from build123d import *

# Parameters (mm, degrees)
SKETCH_3_R               = 275
SKETCH_3_R_2             = 185
SKETCH_3_R_3             = 27
SKETCH_3_R_4             = 18
EXTRUDE_1_DEPTH          = 12
CUT_EXTRUDE_2_DEPTH      = 12
CUT_EXTRUDE_2_DEPTH_BACK = 390.093819021
SKETCH_4_R               = 18


with BuildPart() as part:
    # 草图3 → 凸台-拉伸1 (new body)
    with BuildSketch(Plane(origin=(0, 0, 0), x_dir=(1, 0, 0), z_dir=(0, 1, 0))):
        with Locations(Location((0, 0, 0), (0, 0, 270))):
            Circle(SKETCH_3_R)
        with Locations(Location((0, 0, 0), (0, 0, 270))):
            Circle(SKETCH_3_R_2, mode=Mode.SUBTRACT)
        with Locations(Location((240, 0, 0), (0, 0, 270))):
            Circle(SKETCH_3_R_3, mode=Mode.SUBTRACT)
        with Locations(Location((234.2578125, -52.185029297, 0), (0, 0, 270))):
            Circle(SKETCH_3_R_4, mode=Mode.SUBTRACT)
        with Locations(Location((-120, -207.846096908, 0), (0, 0, 270))):
            Circle(SKETCH_3_R_3, mode=Mode.SUBTRACT)
        with Locations(Location((-120, 207.846096908, 0), (0, 0, 270))):
            Circle(SKETCH_3_R_3, mode=Mode.SUBTRACT)
        with Locations(Location((-71.935345182, 228.965731308, 0), (0, 0, 270))):
            Circle(SKETCH_3_R_4, mode=Mode.SUBTRACT)
        with Locations(Location((-162.322467318, -176.780702012, 0), (0, 0, 270))):
            Circle(SKETCH_3_R_4, mode=Mode.SUBTRACT)
    extrude(amount=EXTRUDE_1_DEPTH)

    # 草图4 → 切除-拉伸2 (cut, two sides: drawn at the far end of the back side and taken through both)
    with BuildSketch(Plane(origin=(0, 0, 0), x_dir=(1, 0, 0), z_dir=(0, 1, 0)).offset(-CUT_EXTRUDE_2_DEPTH_BACK)):
        with Locations(Location((-228, 0, 0), (0, 0, 270))):
            Circle(SKETCH_4_R)
        with Locations(Location((114, 197.453792063, 0), (0, 0, 270))):
            Circle(SKETCH_4_R)
        with Locations(Location((114, -197.453792063, 0), (0, 0, 270))):
            Circle(SKETCH_4_R)
    extrude(amount=CUT_EXTRUDE_2_DEPTH + CUT_EXTRUDE_2_DEPTH_BACK, mode=Mode.SUBTRACT)


solid = part.part
Source: CAD feature listing. Evaluate the final solid. Frame: model axes, mm. Coordinates: 2 decimals unless noted, no trailing zeros. Loops run counter-clockwise (first coordinate to the right, second up) from the corner with the lowest first, then second, coordinate; pieces in that order, holes last. Notation, with made-up numbers: (28, 51.5) - (56, 51.5) arc R13 ccw to (56, 68.5) - close; hole circle Ø4 at (34, -14). An arc over 180 degrees is marked (long way). One line per item, written item: value. Start each with the question number.
1. Section B-B (z = 0). Return the cut outline in (x, y).
2. Mould query, pull axis Z, two halves, no side actions, for faces 1 (the flat face through (-57, 0, 179)), 2 (the cylindrical face through (82.6, 5.9, 262.3)), 3 (the cylindrical face through (-71.14, 5.92, -246.95)). Classes: pulls with the +Z half, pulls with the -Z half, needs draft (parallel to the pull), parting line crosses it, or undercut.
3. Section C-C (x = -120). Return the cut outline in (y, z), and give its area (3 significant figures).
4. Section A-A (x = 0). Return the cut outline in (y, z), and give its area (3 significant figures).
5. Section D-D (z = -160.5). Return the cut outline in (x, y), and give its area (3 significant figures).
6. Contact query for flat-ended pins moving along their axis: P1, Ø4, axis at x = -215.5, y = 6.5, coming from the +Z side; P2, Ø21.5, axis at x = -228, z = 0, coming from the +Y side; P3, Ø1, axis at x = 27.5, y = 10.5, coming from the -Z side; P4, Ø1.5, axis at y = 5, z = 4.5, coming from the +X side. Output: stop coordinate, or through.
7. Ray query, L1, parallel to X at y = 2.5, z = 0; L2, parallel to Z at x = 127.5, y = 9; L3, parallel to X at y = 7.75, z = -201. Return the intervals inside material, ascending.
Verdict:
1. outline: (-275, 0) - (-246, 0) - (-246, 12) - (-275, 12) - close; (-210, 0) - (-185, 0) - (-185, 12) - (-210, 12) - close; (185, 0) - (213, 0) - (213, 12) - (185, 12) - close; (267, 0) - (275, 0) - (275, 12) - (267, 12) - close
2. face 1: needs draft
2. face 2: parting line crosses it
2. face 3: undercut
3. outline: (0, -247.44) - (12, -247.44) - (12, -234.85) - (0, -234.85) - close; (0, -180.85) - (12, -180.85) - (12, -140.8) - (0, -140.8) - close; (0, 140.8) - (12, 140.8) - (12, 180.85) - (0, 180.85) - close; (0, 234.85) - (12, 234.85) - (12, 247.44) - (0, 247.44) - close
3. area: 1,260 mm2
4. outline: (0, -275) - (12, -275) - (12, -185) - (0, -185) - close; (0, 185) - (12, 185) - (12, 275) - (0, 275) - close
4. area: 2,160 mm2
5. outline: (-223.3, 0) - (-92, 0) - (-92, 12) - (-223.3, 12) - close; (92, 0) - (223.3, 0) - (223.3, 12) - (92, 12) - close
5. area: 3,150 mm2
6. P1: stops at z = 173.33
6. P2: passes through
6. P3: stops at z = -273.67
6. P4: stops at x = 274.97
7. L1: x = -275 to -246, -210 to -185, 185 to 213, 267 to 275
7. L2: z = -243.66 to -209.36, -185.55 to -134.05, 134.05 to 185.55, 209.36 to 243.66
7. L3: x = -187.68 to -146.12, -93.88 to 96.35, 131.65 to 187.68
